Here's how the part is built. I have some questions about the finished solid (model axes, mm). Face numbers are marked on the shaded views. A direction names the side the tool comes from. Round coordinates to 2 decimals unless told otherwise and drop trailing zeros.
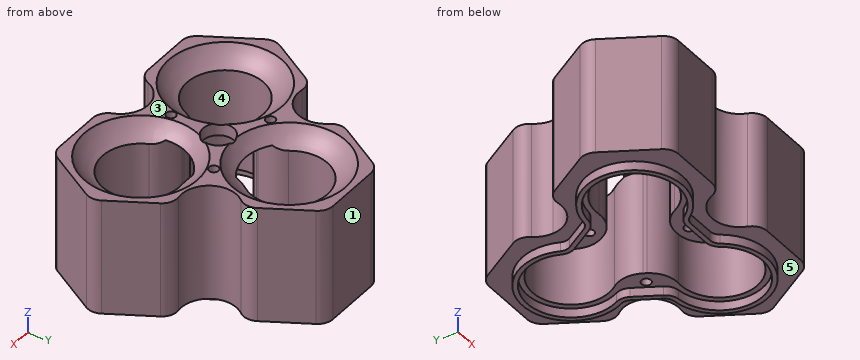
```python
from build123d import *

# Parameters (mm, degrees)
EXTRUDE_3_DEPTH          = 38
SKETCH_1_R               = 6
SKETCH_1_R_2             = 5
CUT_EXTRUDE_2_DEPTH      = 34
PATTERN_CIRCULAR_2_COUNT = 3
SKETCH_1_8_R             = 5
CUT_EXTRUDE_4_DEPTH      = 38
FILLET_2_R               = 5
SKETCH_12_R              = 1.55
CUT_EXTRUDE_5_DEPTH      = 38
SKETCH_17_W              = 6
SKETCH_17_H              = 1.5


with BuildPart() as part:
    # Sketch 8 → Extrude 3 (new body)
    with BuildSketch(Plane.XY):
        with BuildLine():
            Line((11.835680518, 43.594010768), (-11.835680518, 43.594010768))
            Line((-11.835680518, 43.594010768), (-23.253520778, 23.817731326))
            ThreePointArc((-23.253520778, 23.817731326), (-19.959292144, 20.523502692), (-18.753520778, 16.023502692))
            ThreePointArc((-18.753520778, 16.023502692), (-23.253520778, 8.229274058), (-32.253520778, 8.229274058))
            Line((-32.253520778, 8.229274058), (-43.671361037, -11.547005384))
            Line((-43.671361037, -11.547005384), (-31.835680518, -32.047005384))
            Line((-31.835680518, -32.047005384), (-9, -32.047005384))
            ThreePointArc((-9, -32.047005384), (0, -23.047005384), (9, -32.047005384))
            Line((9, -32.047005384), (31.835680518, -32.047005384))
            Line((31.835680518, -32.047005384), (43.671361037, -11.547005384))
            Line((43.671361037, -11.547005384), (32.253520778, 8.229274058))
            ThreePointArc((32.253520778, 8.229274058), (19.959292144, 11.523502692), (23.253520778, 23.817731326))
            Line((23.253520778, 23.817731326), (11.835680518, 43.594010768))
        make_face()
    extrude(amount=EXTRUDE_3_DEPTH)

    # Sketch 1 → Cut-Extrude 2 (cut)
    # profile 1 of 5: a face of its own
    with BuildSketch(Plane.XY):
        with BuildLine():
            Line((-9.762812095, 6.184324194), (-10.237187905, 5.362681189))
            ThreePointArc((-10.237187905, 5.362681189), (-13.893347706, 1.870410777), (-18.855474732, 0.90048681))
            ThreePointArc((-18.855474732, 0.90048681), (-30.825317547, -17.797005384), (-8.647892913, -16.779563523))
            ThreePointArc((-8.647892913, -16.779563523), (-5.326850604, -12.967197446), (-0.47437581, -11.547005384))
            Line((-0.47437581, -11.547005384), (0.47437581, -11.547005384))
            ThreePointArc((0.47437581, -11.547005384), (5.326850604, -12.967197446), (8.647892913, -16.779563523))
            ThreePointArc((8.647892913, -16.779563523), (30.825317547, -17.797005384), (18.855474732, 0.90048681))
            ThreePointArc((18.855474732, 0.90048681), (13.893347706, 1.870410778), (10.237187905, 5.362681189))
            Line((10.237187905, 5.362681189), (9.762812095, 6.184324195))
            ThreePointArc((9.762812095, 6.184324195), (8.566497102, 11.096786669), (10.207581819, 15.879076713))
            ThreePointArc((10.207581819, 15.879076713), (0, 35.594010768), (-10.207581819, 15.879076713))
            ThreePointArc((-10.207581819, 15.879076713), (-8.566497102, 11.096786669), (-9.762812095, 6.184324194))
        make_face()
        with Locations((0, 23.094010768)):
            Circle(SKETCH_1_R, mode=Mode.SUBTRACT)
        with Locations((20, -11.547005384)):
            Circle(SKETCH_1_R, mode=Mode.SUBTRACT)
        with Locations((-20, -11.547005384)):
            Circle(SKETCH_1_R, mode=Mode.SUBTRACT)
    # profile 2 of 5: a face of its own
    with BuildSketch(Plane.XY):
        with Locations((20, -11.547005384)):
            Circle(SKETCH_1_R)
    # profile 3 of 5: a face of its own
    with BuildSketch(Plane.XY):
        with Locations((-20, -11.547005384)):
            Circle(SKETCH_1_R)
    # profile 4 of 5: a face of its own
    with BuildSketch(Plane.XY):
        with Locations((0, 23.094010768)):
            Circle(SKETCH_1_R)
    # profile 5 of 5: a face of its own
    with BuildSketch(Plane.XY):
        Circle(SKETCH_1_R_2)
    extrude(amount=CUT_EXTRUDE_2_DEPTH, mode=Mode.SUBTRACT)

    # Sketch 10 → Cut-Revolve 2 (revolve, cut)
    with BuildSketch(Plane(origin=(0, 0, 0), x_dir=(0, 0, -1), z_dir=(1, 0, 0)), mode=Mode.PRIVATE) as cut_revolve_2_sk:
        with BuildLine():
            Line((-38, 41.594010768), (-38, 23.094010768))
            Line((-38, 23.094010768), (-33, 23.094010768))
            Line((-33, 23.094010768), (-33, 35.594010768))
            ThreePointArc((-33, 35.594010768), (-35.102636282, 38.9251472), (-38, 41.594010768))
        make_face()
    cut_revolve_2 = revolve(cut_revolve_2_sk.sketch.rotate(Axis((0, 23.094010768, 38), (0, 0, -1)), 90), axis=Axis((0, 23.094010768, 38), (0, 0, -1)), mode=Mode.SUBTRACT)

    # Pattern Circular 2: Cut-Revolve 2 ×3 about axis
    pattern_circular_2_axis = Axis((0, 0, 0), (0, 0, 1))
    for i in range(1, PATTERN_CIRCULAR_2_COUNT):
        add(cut_revolve_2.rotate(pattern_circular_2_axis, i * 360 / PATTERN_CIRCULAR_2_COUNT), mode=Mode.SUBTRACT)

    # Sketch 1_8 → Cut-Extrude 4 (cut)
    with BuildSketch(Plane.XY):
        with Locations(Location((0, 0, 0), (0, 0, 189.336379866))):
            Circle(SKETCH_1_8_R)
    extrude(amount=CUT_EXTRUDE_4_DEPTH, mode=Mode.SUBTRACT)

    # Fillet 2
    fillet_2_edges = [part.edges().sort_by_distance(p)[0] for p in [
        (-9, -32.047005384, 19),
        (-31.835680518, -32.047005384, 19),
        (-43.671361037, -11.547005384, 19),
        (-32.253520778, 8.229274058, 19),
        (-23.253520778, 23.817731326, 19),
        (-11.835680518, 43.594010768, 19),
        (11.835680518, 43.594010768, 19),
        (23.253520778, 23.817731326, 19),
        (32.253520778, 8.229274058, 19),
        (43.671361037, -11.547005384, 19),
        (31.835680518, -32.047005384, 19),
        (9, -32.047005384, 19),
    ]]
    fillet(fillet_2_edges, radius=FILLET_2_R)

    # Sketch 12 → Cut-Extrude 5 (cut)
    with BuildSketch(Plane(origin=(0, 0, 0), x_dir=(-1, 0, 0), z_dir=(0, 0, -1))):
        with Locations((-13.423393759, 7.75)):
            Circle(SKETCH_12_R)
        with Locations((13.423393759, 7.75)):
            Circle(SKETCH_12_R)
        with Locations((0, -15.5)):
            Circle(SKETCH_12_R)
    extrude(amount=-CUT_EXTRUDE_5_DEPTH, mode=Mode.SUBTRACT)

    # Sweep 1: sweep along a path in Sketch 13
    with BuildLine(Plane(origin=(0, 0, 0), x_dir=(-1, 0, 0), z_dir=(0, 0, -1))) as sweep_1_path:
        Line((18.316211134, 5.369402481), (13.808144519, 13.177602903))
        ThreePointArc((13.808144519, 13.177602903), (13.276648142, 14.989995098), (13.63598379, 16.844215085))
        ThreePointArc((13.63598379, 16.844215085), (0, 38.094010768), (-13.63598379, 16.844215085))
        ThreePointArc((-13.63598379, 16.844215085), (-13.276648142, 14.989995098), (-13.808144519, 13.177602903))
        Line((-13.808144519, 13.177602903), (-18.316211134, 5.369402481))
        ThreePointArc((-18.316211134, 5.369402481), (-19.620040628, 4.002917019), (-21.405510065, 3.387000825))
        ThreePointArc((-21.405510065, 3.387000825), (-32.990381057, -19.047005384), (-7.769526275, -20.23121591))
        ThreePointArc((-7.769526275, -20.23121591), (-6.343392486, -18.992912117), (-4.508066615, -18.547005384))
        Line((-4.508066615, -18.547005384), (4.508066615, -18.547005384))
        ThreePointArc((4.508066615, -18.547005384), (6.343392486, -18.992912117), (7.769526275, -20.23121591))
        ThreePointArc((7.769526275, -20.23121591), (32.990381057, -19.047005384), (21.405510065, 3.387000825))
        ThreePointArc((21.405510065, 3.387000825), (19.620040628, 4.002917019), (18.316211134, 5.369402481))
    # Sketch 17 → Sweep 1 (sweep)
    with BuildSketch(Plane(origin=(0, 0, 0), x_dir=(0, 0, -1), z_dir=(1, 0, 0))):
        with Locations((0, 38.094010768)):
            Rectangle(SKETCH_17_W, SKETCH_17_H)
    sweep(path=sweep_1_path.line)


solid = part.part
```
1. I'm going to push flat-ended pins straight in: P1, Ø23, axis at x = 20, y = -11.55, coming from the +Z side; P2, Ø12, axis at y = -19.5, z = 15, coming from the -X side; P3, Ø3, axis at x = -26.5, z = 18.5, coming from the +Y side; P4, Ø4, axis at x = -13.42, y = 7.75, coming from the -Z side. Where does each tip first touch, or does it pass through?
Evaluation:
P1: passes through
P2: stops at x = -42.5
P3: stops at y = 7.46
P4: stops at z = 0
2. If we section it at A-A, the plane y = -15.5: State how many separate pieces and enclosed holes the cut face has, and give its area (3 significant figures).
Evaluation:
separate pieces: 4
enclosed holes: 0
area: 1,150 mm2
3. If we mould it in two halves opening along Y, with no side actions, what happens to the marked faces 1, 2 and 3? For each: released by +Y, released by -Y, zero draft, split by the parting line, or undercut.
Evaluation:
face 1: released by +Y
face 2: undercut
face 3: zero draft
4. On a 3-axis mill with a long thin cutter (end or side, diameter ignored), from which of +Z, -Z, +X, -X, +Y, -Y can I reach the whole of each face in a straight line? I mean the marked faces 4 and 5. Say none if no direction works.
Evaluation:
face 4: +Z, -Z
face 5: -Z
5. I need wall thicknesses on probe 1 along Y at (x, z) = (20, 17); probe 2 along X at (y, z) = (29.5, 29); probe 3 along Y at (x, z) = (14, 4). Which ranges of each line are inside material? Lowest first, please.
Evaluation:
probe 1: y = -32.05 to -24.05, 0.95 to 11.45, 20.59 to 29.45
probe 2: x = -19.97 to -10.73, 10.73 to 19.97
probe 3: y = -32.05 to -22.51, 1.82 to 6.31, 9.19 to 39.85
